from build123d import *

# Parameters (mm, degrees)
BOSS_EXTRUDE1_DEPTH = 15
FILLET1_R           = 2


with BuildPart() as part:
    # Sketch1 → Boss-Extrude1 (new body)
    with BuildSketch(Plane.XY):
        with BuildLine():
            Line((0, 0), (0, 15.5))
            Line((0, 15.5), (119, 15.5))
            ThreePointArc((119, 15.5), (119.707106781, 15.792893219), (120, 16.5))
            Line((120, 16.5), (120, 17))
            ThreePointArc((120, 17), (119.707106781, 17.707106781), (119, 18))
            Line((119, 18), (-2.5, 18))
            Line((-2.5, 18), (-2.5, -2.5))
            Line((-2.5, -2.5), (119, -2.5))
            ThreePointArc((119, -2.5), (119.707106781, -2.207106781), (120, -1.5))
            Line((120, -1.5), (120, -1))
            ThreePointArc((120, -1), (119.707106781, -0.292893219), (119, 0))
            Line((119, 0), (0, 0))
        make_face()
    extrude(amount=BOSS_EXTRUDE1_DEPTH)

    # Fillet1
    fillet1_edges = [part.edges().sort_by_distance(p)[0] for p in [
        (0, 15.5, 7.5),
        (0, 0, 7.5),
    ]]
    fillet(fillet1_edges, radius=FILLET1_R)


solid = part.part
For this review, take the finished solid that the model builds, in its own axes (mm). A direction names the side the tool comes from. Give positions to 0.01 mm unless a question says otherwise; leave off trailing zeros. Loops run counter-clockwise (first coordinate to the right, second up) from the corner with the lowest first, then second, coordinate; pieces in that order, holes last.
Item 1: Draft analysis for pull direction Y (two halves, no side actions). For faces 3 (the cylindrical face through (0.57, 0.6, 7.6)), 4 (the flat face through (49, -1, 15)), 5 (the flat face through (59, 18, 7)), state which applies: +Y half, -Y half, draft (parallel to the pull), parting line (faces both ways), or undercut.
Item 2: Insertion check: pin 1 (6 mm diameter, centred on y = 6, z = 9, fed in from +X). The pin has a flat end and moves straight along its axis. Give the tip position at first contact, or say it passes through.
Item 3: Take a section at A-A, the plane x = 71. State the section outline as (y, z) points, and give its area (3 significant figures).
Item 4: For line 1 along Y through (x, z) = (90.5, 1); line 2 along X through (y, z) = (3.75, 2); line 3 along X through (y, z) = (15, 1.25), list the stretches that pass through material, from the lowest coordinate up.
Item 5: Take a section at B-B, the plane z = 12.5. State the section outline as (x, y) points.
Item 6: Tool access review of faces 1 (the flat face through (0, 8, 7)), 2 (the flat face through (-2.5, 8, 7)): name each direction out of +Z, -Z, +X, -X, +Y, -Y from which nothing blocks a thin tool from reaching the whole face with its end or side.
Item 7: Take a section at C-C, the plane y = 6.75. State the section outline as (x, z) points, and give its area (3 significant figures).
Calculated:
1. face 3: undercut
1. face 4: draft
1. face 5: +Y half
2. pin 1: stops at x = 0
3. outline: (-2.5, 0) - (0, 0) - (0, 15) - (-2.5, 15) - close; (15.5, 0) - (18, 0) - (18, 15) - (15.5, 15) - close
3. area: 75.0 mm2
4. line 1: y = -2.5 to 0, 15.5 to 18
4. line 2: x = -2.5 to 0
4. line 3: x = -2.5 to 0.68
5. outline: (-2.5, -2.5) - (119, -2.5) arc R1 ccw to (120, -1.5) - (120, -1) arc R1 ccw to (119, 0) - (2, 0) arc R2 cw to (0, 2) - (0, 13.5) arc R2 cw to (2, 15.5) - (119, 15.5) arc R1 ccw to (120, 16.5) - (120, 17) arc R1 ccw to (119, 18) - (-2.5, 18) - close
6. face 1: +Z, -Z, +X
6. face 2: +Z, -Z, -X, +Y, -Y
7. outline: (-2.5, 0) - (0, 0) - (0, 15) - (-2.5, 15) - close
7. area: 37.5 mm2
